Here's the drawing with two shaded views (mm, measured from the low corner). I have some questions. Round coordinates to 2 decimals unless told otherwise and drop trailing zeros. Loops run counter-clockwise (first coordinate to the right, second up) from the corner with the lowest first, then second, coordinate; pieces in that order, holes last. Notation, with made-up numbers: M -19.75,-19 L 13.25,-19 A17 ccw 13.25,-3 Z; hole C 85.5,0 d4. An arc over 180 degrees is marked long. Answer as a JSON object with one key per item and string values.
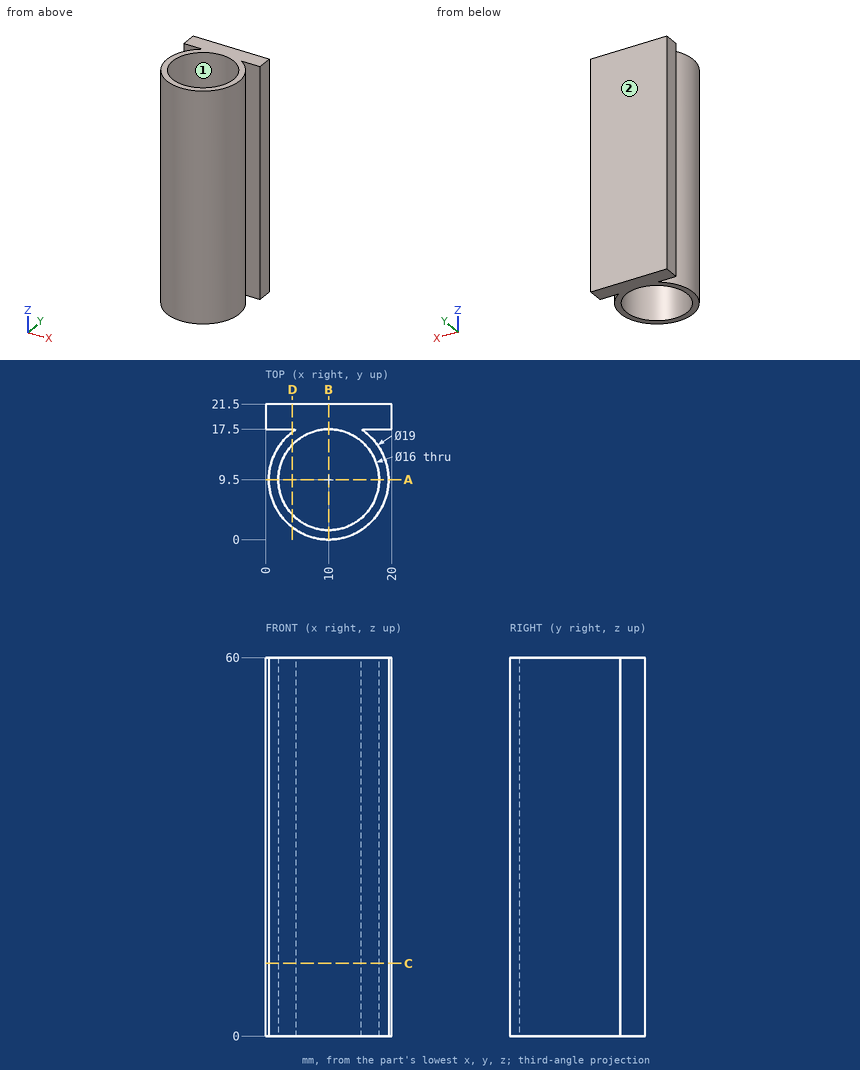
Item 1: We'd pull the mould along X, two halves only. Please class the marked faces 1 and 2: +X half, -X half, draft (parallel to the pull), parting line (faces both ways), or undercut.
Solution:
{"face 1": "undercut", "face 2": "draft"}
Item 2: I want a section at B-B on x = 10. List the corners of the cut face in (y, z) for me.
Solution:
{"outline": "M 0,0 L 1.5,0 L 1.5,60 L 0,60 Z; M 17.5,0 L 21.5,0 L 21.5,60 L 17.5,60 Z"}
Item 3: I want a section at A-A on y = 9.5. List the corners of the cut face in (x, z) for me, plus the area to 3 significant figures.
Solution:
{"outline": "M 0.5,0 L 2,0 L 2,60 L 0.5,60 Z; M 18,0 L 19.5,0 L 19.5,60 L 18,60 Z", "area": "180 mm2"}
Item 4: If I drill on L1, parallel to X at y = 9.5, z = 38; L2, parallel to Y at x = 10, z = 13; L3, parallel to Y at x = 15.75, z = 8, over which ranges is the centre line in solid material (lowest first)? Write a range as from..to.
Solution:
{"L1": "x = 0.5..2, 18..19.5", "L2": "y = 0..1.5, 17.5..21.5", "L3": "y = 1.94..3.94, 15.06..17.06, 17.5..21.5"}
Item 5: For P1, Ø3, axis at y = 3.5, z = 42, coming from the +X side; P2, Ø8, axis at y = 10.5, z = 32.5, coming from the -X side; P3, Ø5.5, axis at x = 18.5, z = 21, coming from the -Y side, each with a flat end and sliding along its axis, tell me the tip position at first contact or that it passes through.
Solution:
{"P1": "stops at x = 18.37", "P2": "stops at x = 0.5", "P3": "stops at y = 1.94"}
Item 6: I want a section at C-C on z = 11.5. List the corners of the cut face in (x, y) for me.
Solution:
{"outline": "M 0,17.5 L 4.88,17.5 A9.5 ccw long 15.12,17.5 L 20,17.5 L 20,21.5 L 0,21.5 Z; hole C 10,9.5 d16"}
Item 7: I want a section at D-D on x = 4.25. List the corners of the cut face in (y, z) for me, plus the area to 3 significant figures.
Solution:
{"outline": "M 1.94,0 L 3.94,0 L 3.94,60 L 1.94,60 Z; M 15.06,0 L 17.06,0 L 17.06,60 L 15.06,60 Z; M 17.5,0 L 21.5,0 L 21.5,60 L 17.5,60 Z", "area": "480 mm2"}
